```python
from build123d import *

# Parameters (mm, degrees)
F0_W     = 8
F0_H     = 5
F1_DEPTH = 8
F2_R     = 1.25
F3_DEPTH = 1.5
F4_DEPTH = 1.5
F5_R     = 0.425
F6_DEPTH = 25
F7_DEPTH = 25


with BuildPart() as f1:
    # F0 (on Front) → F1 (new body)
    with BuildSketch(Plane.XZ):
        with Locations((-1.863892, 2.5)):
            Rectangle(F0_W, F0_H)
    extrude(amount=F1_DEPTH)

    # F2 (on face) → F3 (cut)
    with BuildSketch(Plane.XZ.offset(8)):
        with Locations((-3.863892, 2.5)):
            Circle(F2_R)
    extrude(amount=-F3_DEPTH, mode=Mode.SUBTRACT)

    # F2 (on face) → F4 (cut)
    with BuildSketch(Plane.XZ.offset(8)):
        with Locations((0.136108, 2.5)):
            Circle(F2_R)
    extrude(amount=-F4_DEPTH, mode=Mode.SUBTRACT)

    # F5 (on face) → F6 (cut)
    with BuildSketch(Plane.XZ.offset(8)):
        with Locations((0.136108, 2.5)):
            Circle(F5_R)
    extrude(amount=-F6_DEPTH, mode=Mode.SUBTRACT)

    # F5 (on face) → F7 (cut)
    with BuildSketch(Plane.XZ.offset(8)):
        with Locations((-3.863892, 2.5)):
            Circle(F5_R)
        with Locations((0.136108, 2.5)):
            Circle(F5_R)
    extrude(amount=-F7_DEPTH, mode=Mode.SUBTRACT)


solid = f1.part
```
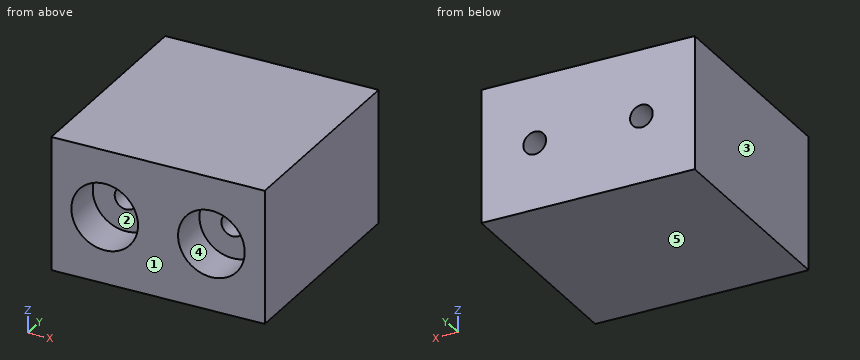
Input: part model. Units: mm. Frame: model coordinates. Face numbers are marked on the shaded views. A direction names the side the tool comes from. Round coordinates to 2 decimals unless told otherwise and drop trailing zeros. Loops run counter-clockwise (first coordinate to the right, second up) from the corner with the lowest first, then second, coordinate; pieces in that order, holes last.
1) Section query A-A on z = 2.5. Return the cut outline in (x, y), plus the area to 4 significant figures.
Ans:
outline: (-5.86, -8) - (-5.11, -8) - (-5.11, -6.5) - (-4.29, -6.5) - (-4.29, 0) - (-5.86, 0) - close; (-3.44, -6.5) - (-2.61, -6.5) - (-2.61, -8) - (-1.11, -8) - (-1.11, -6.5) - (-0.29, -6.5) - (-0.29, 0) - (-3.44, 0) - close; (0.56, -6.5) - (1.39, -6.5) - (1.39, -8) - (2.14, -8) - (2.14, 0) - (0.56, 0) - close
area: 45.45 mm2
2) Pin query (flat end, axial travel): pin 1 (0.8 mm diameter, centred on x = 0.5, z = 2.5, fed in from -Y). Return the tip coordinate at first contact, or that it passes through.
Ans:
pin 1: stops at y = -6.5
3) Section query C-C on z = 1.5. Return the cut outline in (x, y), plus the area to 3 significant figures.
Ans:
outline: (-5.86, -8) - (-4.61, -8) - (-4.61, -6.5) - (-3.11, -6.5) - (-3.11, -8) - (-0.61, -8) - (-0.61, -6.5) - (0.89, -6.5) - (0.89, -8) - (2.14, -8) - (2.14, 0) - (-5.86, 0) - close
area: 59.5 mm2
4) Set-up query: the marked faces 4 and 5. Return all of +Z, -Z, +X, -X, +Y, -Y with unobstructed straight access to the full face (end or side cutting, diameter ignored); none if empty.
Ans:
face 4: -Y
face 5: -Z, +X, -X, +Y, -Y
5) Pull-direction query (X, two-part tool) for the marked faces 1, 2 and 3; classes: released by +X, released by -X, zero draft, split by the parting line, or undercut.
Ans:
face 1: zero draft
face 2: undercut
face 3: released by -X
6) Material intervals for line 1 (Y direction, x = -5, z = 2.25); line 2 (Z direction, x = 0, y = -5.5), sorted ascending.
Ans:
line 1: y = -6.5 to 0
line 2: z = 0 to 2.1, 2.9 to 5
7) Section query B-B on y = -3.75. Return the cut outline in (x, z) (3 decimals), plus the area to 3 significant figures.
Ans:
outline: (-5.864, 0) - (2.136, 0) - (2.136, 5) - (-5.864, 5) - close; hole circle Ø0.85 at (-3.864, 2.5); hole circle Ø0.85 at (0.136, 2.5)
area: 38.9 mm2
